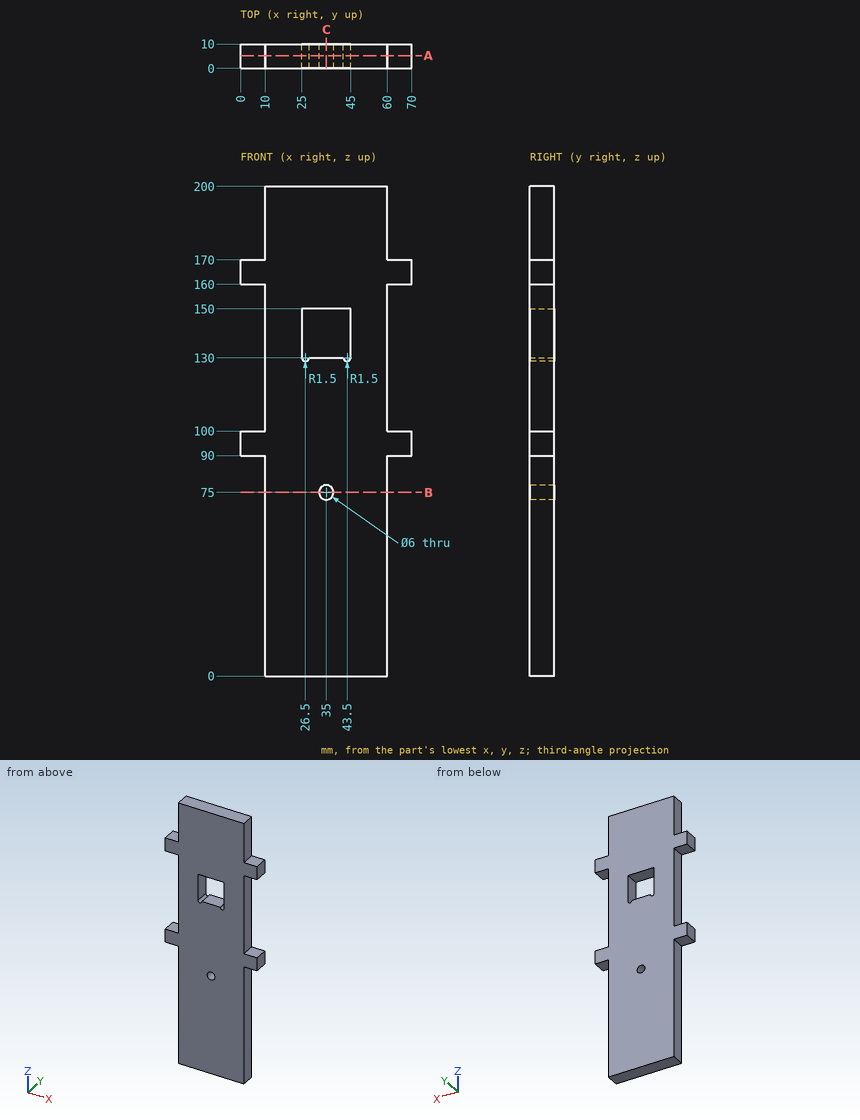
Job drawing, mm, ordinate dimensions from the low corner. One solid piece. Round coordinates to 2 decimals unless told otherwise and drop trailing zeros. Order: outer loops, then holes, each group sorted by start corner. A loop starts at its lowest first (then second) coordinate and runs counter-clockwise, first axis right, second up. Notation, with made-up numbers: (24.5, -23.5) -> (30.5, -23.5) arc R19 ccw to (30.5, -19.5) -> close; hole circle Ø7 at (-25, 11.25). An arc over 180 degrees is marked (long way). Answer in a Markdown table with one row per item.
1) Wall check: L1, parallel to Z at x = 35, y = 2.75; L2, parallel to Z at x = 30, y = 9.75; L3, parallel to X at y = 8.5, z = 132.5. Give the ranges that are in metal, low to high.
Values:
| item | result |
|---|---|
| L1 | 0 to 72, 78 to 130, 150 to 200 |
| L2 | 0 to 130, 150 to 200 |
| L3 | 10 to 25, 45 to 60 |
2) Band-saw the part on A-A on y = 5.25. Give the cut face in (x, z).
Values:
| item | result |
|---|---|
| outline | (0, 90) -> (10, 90) -> (10, 0) -> (60, 0) -> (60, 90) -> (70, 90) -> (70, 100) -> (60, 100) -> (60, 160) -> (70, 160) -> (70, 170) -> (60, 170) -> (60, 200) -> (10, 200) -> (10, 170) -> (0, 170) -> (0, 160) -> (10, 160) -> (10, 100) -> (0, 100) -> close; hole (25, 130) arc R1.5 ccw to (28, 130) -> (42, 130) arc R1.5 ccw to (45, 130) -> (45, 150) -> (25, 150) -> close; hole circle Ø6 at (35, 75) |
3) Band-saw the part on B-B on z = 75. Give the cut face in (x, y), and give its area (3 significant figures).
Values:
| item | result |
|---|---|
| outline | (10, 0) -> (32, 0) -> (32, 10) -> (10, 10) -> close; (38, 0) -> (60, 0) -> (60, 10) -> (38, 10) -> close |
| area | 440 mm2 |
4) Band-saw the part on C-C on x = 35. Give the cut face in (y, z), and give its area (3 significant figures).
Values:
| item | result |
|---|---|
| outline | (0, 0) -> (10, 0) -> (10, 72) -> (0, 72) -> close; (0, 78) -> (10, 78) -> (10, 130) -> (0, 130) -> close; (0, 150) -> (10, 150) -> (10, 200) -> (0, 200) -> close |
| area | 1,740 mm2 |
5) Pin check, flat tips, straight feed: P1, Ø3, axis at x = 5, y = 6, coming from the -Z side; P2, Ø3, axis at x = 6, y = 7, coming from the +Z side; P3, Ø3, axis at y = 2.5, z = 142, coming from the +X side. Stop position of each tip, or through.
Values:
| item | result |
|---|---|
| P1 | z = 90 |
| P2 | z = 170 |
| P3 | x = 60 |
